```python
from build123d import *

# Parameters (mm, degrees)
SKETCH_R        = 17.5
SKETCH_R_2      = 8.05
SKETCH_R_3      = 2.6
PAD_DEPTH       = 5.2
SKETCH001_R     = 8.05
PAD001_DEPTH    = 0.2
CHAMFER001_SIZE = 0.25


with BuildPart() as part:
    # Sketch → Pad (new body)
    with BuildSketch(Plane.XY):
        Circle(SKETCH_R)
        Circle(SKETCH_R_2, mode=Mode.SUBTRACT)
        with Locations((12.5, 0)):
            Circle(SKETCH_R_3, mode=Mode.SUBTRACT)
        with Locations((-12.5, 0)):
            Circle(SKETCH_R_3, mode=Mode.SUBTRACT)
        with Locations((-6.25, 10.825318)):
            Circle(SKETCH_R_3, mode=Mode.SUBTRACT)
        with Locations((6.25, 10.825318)):
            Circle(SKETCH_R_3, mode=Mode.SUBTRACT)
        with Locations((-6.25, -10.825318)):
            Circle(SKETCH_R_3, mode=Mode.SUBTRACT)
        with Locations((6.25, -10.825318)):
            Circle(SKETCH_R_3, mode=Mode.SUBTRACT)
    extrude(amount=PAD_DEPTH)

    # Sketch001 → Pad001 (join)
    with BuildSketch(Plane.XY):
        with BuildLine():
            ThreePointArc((0, 17.5), (-17.5, 0), (0, -17.5))
            Line((0, -17.5), (0, -25))
            ThreePointArc((0, -25), (25, 0), (0, 25))
            Line((0, 17.5), (0, 25))
        make_face()
        Circle(SKETCH001_R, mode=Mode.SUBTRACT)
    extrude(amount=PAD001_DEPTH)

    # Chamfer001
    chamfer001_edges = [part.edges().sort_by_distance(p)[0] for p in [
        (-17.5, 0, 5.2),
        (-8.05, 0, 5.2),
        (3.65, -10.825318, 5.2),
        (-8.85, 10.825318, 5.2),
        (-15.1, 0, 5.2),
        (9.9, 0, 5.2),
        (-8.85, -10.825318, 5.2),
        (3.65, 10.825318, 5.2),
    ]]
    chamfer(chamfer001_edges, length=CHAMFER001_SIZE)


solid = part.part
```
CAD build for the part. Positions are in the model's coordinates, mm. A direction names the side the tool comes from. Coordinates: 2 decimals unless noted, no trailing zeros. Order: outer loops, then holes, each group sorted by start corner. A loop starts at its lowest first (then second) coordinate and runs counter-clockwise, first axis right, second up. Notation, with made-up numbers: M 82.25,-4 L 141.25,-4 A16 cw 141.25,14 Z; hole C -27,71 d8. An arc over 180 degrees is marked long. Answer as CSV lines item,"result".
1) Flat gauge pins, fed straight in: P1, Ø1.5, axis at y = 4, z = 2.5, coming from the +X side; P2, Ø2.5, axis at x = -12, y = -0.5, coming from the +Z side; P3, Ø1, axis at y = -3, z = 1, coming from the -X side; P4, Ø13, axis at x = 0, y = 0, coming from the -Z side. Where does each tip first touch, or does it go through?
Verdict:
P1,"x = 17.2"
P2,"z = 0.2"
P3,"x = -17.32"
P4,"through"
2) 3-axis set-ups, long thin cutter, end or side, ignore diameter. For faces 4 (the cylindrical face through (-10.02, 0.78, 2.54)), 5 (the flat face through (-4.1, -7.4, 5.2)): which of +Z, -Z, +X, -X, +Y, -Y reach the whole face in a straight line?
Verdict:
face 4,"+Z"
face 5,"+Z, +X, -X, +Y, -Y"
3) Drill centre lines: L1, parallel to X at y = -13, z = 2.15; L2, parallel to X at y = -1, z = 3.05; L3, parallel to Y at x = 0, z = 3. Where is each one in solid material? Low to high. Write a range as from..to.
Verdict:
L1,"-11.72..-7.68, -4.82..4.82, 7.68..11.72"
L2,"-17.47..-14.9, -10.1..-7.99, 7.99..10.1, 14.9..17.47"
L3,"-17.5..-8.05, 8.05..17.5"
4) Mould opens along X. For faces 1 (the flat face through (-6, -11, 0.2)), 2 (the cylindrical face through (14.98, 0.78, 2.54)), 3 (the flat face through (18, 0, 0.2)) say: released by +X, released by -X, zero draft, split by the parting line, or undercut.
Verdict:
face 1,"undercut"
face 2,"undercut"
face 3,"zero draft"
5) Cut at C-C (y = 18.5). List the corners of the cut face in (x, z).
Verdict:
outline,"M 0,0 L 16.82,0 L 16.82,0.2 L 0,0.2 Z"
6) Cut at B-B (z = 4.1). List the corners of the cut face in (x, y).
Verdict:
outline,"C 0,0 d35; hole C -12.5,0 d5.2; hole C -6.25,-10.83 d5.2; hole C -6.25,10.83 d5.2; hole C 0,0 d16.1; hole C 6.25,-10.83 d5.2; hole C 6.25,10.83 d5.2; hole C 12.5,0 d5.2"
7) Cut at A-A (y = 0). List the corners of the cut face in (x, z), then the cut area to 3 significant figures.
Verdict:
outline,"M -17.5,0 L -8.05,0 L -8.05,4.95 L -8.3,5.2 L -9.65,5.2 L -9.9,4.95 L -9.9,0.2 L -15.1,0.2 L -15.1,4.95 L -15.35,5.2 L -17.25,5.2 L -17.5,4.95 Z; M 8.05,0 L 25,0 L 25,0.2 L 17.5,0.2 L 17.5,4.95 L 17.25,5.2 L 15.35,5.2 L 15.1,4.95 L 15.1,0.2 L 9.9,0.2 L 9.9,4.95 L 9.65,5.2 L 8.3,5.2 L 8.05,4.95 Z"
area,"47.5 mm2"
